from build123d import *

# Parameters (mm, degrees)
SKETCH1_W                 = 20
SKETCH1_H                 = 45
BOSS_EXTRUDE1_DEPTH       = 30
SKETCH2_R                 = 1.5
BOSS_EXTRUDE2_DEPTH       = 7
F_4_48_TAPPED_HOLE1_D     = 2.3749
F_4_48_TAPPED_HOLE1_DEPTH = 3.5
F_4_48_TAPPED_HOLE1_TIP   = 0.713491942


with BuildPart() as part:
    # Sketch1 → Boss-Extrude1 (new body)
    with BuildSketch(Plane(origin=(0, 0, 0), x_dir=(1, 0, 0), z_dir=(0, 1, 0))):
        Rectangle(SKETCH1_W, SKETCH1_H)
    extrude(amount=BOSS_EXTRUDE1_DEPTH)

    # Sketch2 → Boss-Extrude2 (add)
    with BuildSketch(Plane(origin=(0, 30, 0), x_dir=(1, 0, 0), z_dir=(0, 1, 0))):
        with Locations((0, 12.5)):
            Circle(SKETCH2_R)
    extrude(amount=BOSS_EXTRUDE2_DEPTH)

    # #4-48 Tapped Hole1
    with Locations(Plane.ZY.offset(10)):
        with Locations((-12.8, 7.5), (-12.8, 22.5), (14.5, 22.5), (14.5, 7.5)):
            Hole(F_4_48_TAPPED_HOLE1_D / 2, depth=F_4_48_TAPPED_HOLE1_DEPTH)
            with Locations((0, 0, -(F_4_48_TAPPED_HOLE1_DEPTH + F_4_48_TAPPED_HOLE1_TIP / 2))):  # 118° drill point
                Cone(0, F_4_48_TAPPED_HOLE1_D / 2, F_4_48_TAPPED_HOLE1_TIP, mode=Mode.SUBTRACT)


solid = part.part
Source: CAD feature listing. Evaluate the final solid. Frame: model axes, mm. A direction names the side the tool comes from. Round coordinates to 2 decimals unless told otherwise and drop trailing zeros. Loops run counter-clockwise (first coordinate to the right, second up) from the corner with the lowest first, then second, coordinate; pieces in that order, holes last. Notation, with made-up numbers: (9, 48.5) -> (18, 48.5) arc R36 ccw to (18, 87.5) -> close; hole circle Ø1 at (9, 58.25). An arc over 180 degrees is marked (long way). Answer as a JSON object with one key per item and string values. Group by question number.
Q1. Mould query, pull axis Z, two halves, no side actions, for faces 4 (the flat face through (0, 30, 0)), 5 (the flat face through (0, 15, -22.5)), 6 (the cylindrical face through (-8.23, 22.86, -13.93)). Classes: pulls with the +Z half, pulls with the -Z half, needs draft (parallel to the pull), parting line crosses it, or undercut.
Q2. Contact query for flat-ended pins moving along their axis: P1, Ø6, axis at x = 4, z = -9, coming from the +Y side; P2, Ø1.4, axis at y = 7.5, z = 14.5, coming from the -X side. Output: stop coordinate, or through.
Q3. Section query B-B (x = 0). Output: boundary loops of the cut face in (y, z), plus the area to 3 significant figures.
Q4. Access query for faces 1 (the cylindrical face through (0, 33, -11)), 2 (the flat face through (-10, 15, 0)), 3 (the cylindrical face through (-8.226, 6.777, 15.442)). Directions: +Z, -Z, +X, -X, +Y, -Y. A direction counts if a zero-diameter tool reaches every point of the face in a straight line with its end or side. Return the directions, or none.
Q5. Ray query, line 1 (Z direction, x = -7.75, y = 7.5); line 2 (Y direction, x = -8.55, z = 14.5); line 3 (Y direction, x = 3.25, z = -10.5). Return the intervals inside material, ascending. Write a range as from..to.
Q6. Section query A-A (x = -7). Output: boundary loops of the cut face in (y, z).
Q7. Section query C-C (z = -8). Output: boundary loops of the cut face in (x, y).
Q8. Section query D-D (y = 34). Output: boundary loops of the cut face in (x, z), plus the area to 3 significant figures.
Completed:
{
 "1": {"face 4": "needs draft", "face 5": "pulls with the -Z half", "face 6": "undercut"},
 "2": {"P1": "y = 30", "P2": "x = -6.21"},
 "3": {"outline": "(0, -22.5) -> (30, -22.5) -> (30, -14) -> (37, -14) -> (37, -11) -> (30, -11) -> (30, 22.5) -> (0, 22.5) -> close", "area": "1,370 mm²"},
 "4": {"face 1": "+Y", "face 2": "+Z, -Z, -X, +Y, -Y", "face 3": "-X"},
 "5": {"line 1": "-22.5..-13.99, -11.61..13.31, 15.69..22.5", "line 2": "0..6.31, 8.69..21.31, 23.69..30", "line 3": "0..30"},
 "6": {"outline": "(0, -22.5) -> (30, -22.5) -> (30, 22.5) -> (0, 22.5) -> close; hole circle Ø2.37 at (7.5, -12.8); hole circle Ø2.37 at (7.5, 14.5); hole circle Ø2.37 at (22.5, -12.8); hole circle Ø2.37 at (22.5, 14.5)"},
 "7": {"outline": "(-10, 0) -> (10, 0) -> (10, 30) -> (-10, 30) -> close"},
 "8": {"outline": "circle Ø3 at (0, -12.5)", "area": "7.07 mm²"}
}
